CAD build for the part. Positions are in the model's coordinates, mm. Face numbers are marked on the shaded views. A direction names the side the tool comes from. Round coordinates to 2 decimals unless told otherwise and drop trailing zeros. Loops run counter-clockwise (first coordinate to the right, second up) from the corner with the lowest first, then second, coordinate; pieces in that order, holes last. Notation, with made-up numbers: M 53,59 L 107,59 A26 cw 107,77 Z; hole C 26.25,12.5 d4. An arc over 180 degrees is marked long. Use a Markdown table: item, result. Add a question column.
(1) Band-saw the part on D-D, the plane y = 25. Write the cut outline in (x, z), and give its area (3 significant figures).
(2) Which spindle directions (+Z, -Z, +X, -X, +Y, -Y) get a long thin tool onto all of the face, cutting with end or side? Do the marked faces 5, 6 and 7. Say none if no direction does.
(3) Band-saw the part on C-C, the plane x = 22.5. Write the cut outline in (y, z).
(4) Flat gauge pins, fed straight in: P1, Ø1.5, axis at y = 43, z = 27, coming from the +X side; P2, Ø6, axis at x = 74.5, y = 7.5, coming from the +Z side. Where does each tip first touch, or does it go through?
(5) Band-saw the part on A-A, the plane z = 40. Write the cut outline in (x, y), and give its area (3 significant figures).
(6) Band-saw the part on B-B, the plane z = 24. Write the cut outline in (x, y), and give its area (3 significant figures).
(7) Wall check: L1, parallel to Z at x = 3, y = 25; L2, parallel to X at y = 17.5, z = 22; L3, parallel to Y at x = 22.5, z = 65.75. Give the ranges that are in metal, low to high.
(8) Two-plate mould, pull along Y, no slides. Class the marked faces 1, 2, 3 and 4: released by +Y, released by -Y, zero draft, split by the parting line, or undercut.
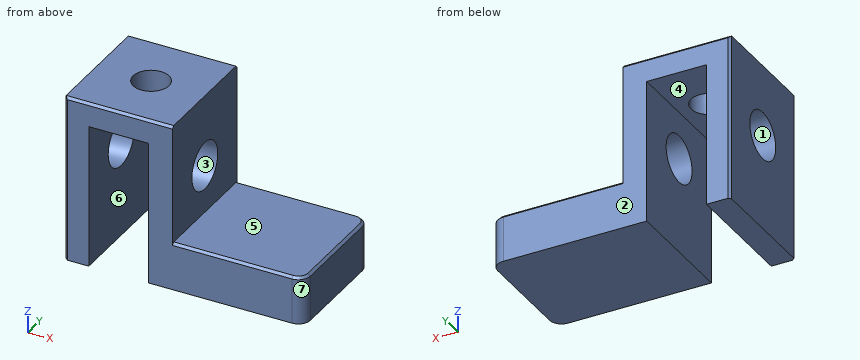
from build123d import *

# Parameters (mm, degrees)
F0_W     = 100
F0_H     = 50
F1_DEPTH = 20
F2_W     = 45
F2_H     = 50
F3_DEPTH = 50
F4_W     = 25
F4_H     = 60
F5_DEPTH = 50.001
F6_R     = 10
F7_DEPTH = 100.001
F8_R     = 7.5
F9_DEPTH = 10
F10_R    = 5
F11_SIZE = 1


with BuildPart() as f1:
    # F0 (on Top) → F1 (new body)
    with BuildSketch(Plane.XY):
        with Locations((50, 25)):
            Rectangle(F0_W, F0_H)
    extrude(amount=F1_DEPTH)

    # F2 (on face) → F3 (join)
    with BuildSketch(Plane.XY.offset(20)):
        with Locations((22.5, 25)):
            Rectangle(F2_W, F2_H)
    extrude(amount=F3_DEPTH)

    # F4 (on face) → F5 (cut, through all)
    with BuildSketch(Plane.XZ):
        with Locations((22.5, 30)):
            Rectangle(F4_W, F4_H)
    extrude(amount=-F5_DEPTH, mode=Mode.SUBTRACT)

    # F6 (on face) → F7 (cut, through all)
    with BuildSketch(Plane(origin=(0, 0, 0), x_dir=(0, -1, 0), z_dir=(-1, 0, 0))):
        with Locations((-25, 40)):
            Circle(F6_R)
    extrude(amount=-F7_DEPTH, mode=Mode.SUBTRACT)

    # F8 (on face) → F9 (cut, through all)
    with BuildSketch(Plane.XY.offset(70)):
        with Locations((22.5, 25)):
            Circle(F8_R)
    extrude(amount=-F9_DEPTH, mode=Mode.SUBTRACT)

    # F10
    f10_edges = [f1.edges().sort_by_distance(p)[0] for p in [
        (100, 0, 10),
        (100, 50, 10),
    ]]
    fillet(f10_edges, radius=F10_R)

    # F11
    f11_edges = [f1.edges().sort_by_distance(p)[0] for p in [
        (0, 0, 35),
        (22.5, 0, 70),
        (0, 50, 35),
        (22.5, 50, 70),
        (70, 50, 20),
        (70, 0, 20),
    ]]
    chamfer(f11_edges, length=F11_SIZE)


solid = f1.part
Return value:
| question | item | result |
|---|---|---|
| 1 | outline | M 0,0 L 10,0 L 10,30 L 0,30 Z; M 0,50 L 10,50 L 10,60 L 15,60 L 15,70 L 0,70 Z; M 30,60 L 35,60 L 35,50 L 45,50 L 45,70 L 30,70 Z; M 35,0 L 100,0 L 100,19 L 99,20 L 45,20 L 45,30 L 35,30 Z |
| 1 | area | 2,200 mm^2 |
| 2 | face 5 | +Z, +X, +Y, -Y |
| 2 | face 6 | -Z, +Y, -Y |
| 2 | face 7 | +Z, -Z, +X, -Y |
| 3 | outline | M 0,60 L 17.5,60 L 17.5,70 L 1,70 L 0,69 Z; M 32.5,60 L 50,60 L 50,69 L 49,70 L 32.5,70 Z |
| 4 | P1 | x = 45 |
| 4 | P2 | z = 20 |
| 5 | outline | M 0,1 L 1,0 L 10,0 L 10,15 L 0,15 Z; M 0,35 L 10,35 L 10,50 L 1,50 L 0,49 Z; M 35,0 L 45,0 L 45,15 L 35,15 Z; M 35,35 L 45,35 L 45,50 L 35,50 Z |
| 5 | area | 599 mm^2 |
| 6 | outline | M 0,1 L 1,0 L 10,0 L 10,50 L 1,50 L 0,49 Z; M 35,0 L 45,0 L 45,50 L 35,50 Z |
| 6 | area | 999 mm^2 |
| 7 | L1 | 0 to 30, 50 to 70 |
| 7 | L2 | 0 to 10, 35 to 45 |
| 7 | L3 | 0 to 17.5, 32.5 to 50 |
| 8 | face 1 | undercut |
| 8 | face 2 | released by +Y |
| 8 | face 3 | undercut |
| 8 | face 4 | zero draft |
